```python
from build123d import *

# Parameters (mm, degrees)
SKETCH1_W           = 59.6
SKETCH1_H           = 35.5
BOSS_EXTRUDE1_DEPTH = 2.5
SKETCH3_W           = 59.6
SKETCH3_H           = 35.5
SKETCH3_W_2         = 54.6
SKETCH3_H_2         = 30.5
BOSS_EXTRUDE4_DEPTH = 38.5
SKETCH4_W           = 3.2
SKETCH4_H           = 3.2
SKETCH4_R           = 0.5
BOSS_EXTRUDE7_DEPTH = 5
FILLET1_R           = 0.25
FILLET2_R           = 0.25
SKETCH6_R           = 2
CUT_EXTRUDE1_DEPTH  = 5
FILLET4_R           = 0.3


with BuildPart() as part:
    # Sketch1 → Boss-Extrude1 (new body)
    with BuildSketch(Plane(origin=(0, 0, 0), x_dir=(1, 0, 0), z_dir=(0, 1, 0))):
        Rectangle(SKETCH1_W, SKETCH1_H)
    extrude(amount=BOSS_EXTRUDE1_DEPTH)

    # Sketch3 → Boss-Extrude4 (add)
    with BuildSketch(Plane(origin=(0, 2.5, 0), x_dir=(1, 0, 0), z_dir=(0, 1, 0))):
        Rectangle(SKETCH3_W, SKETCH3_H)
        Rectangle(SKETCH3_W_2, SKETCH3_H_2, mode=Mode.SUBTRACT)
    extrude(amount=BOSS_EXTRUDE4_DEPTH)

    # Sketch4 → Boss-Extrude7 (add)
    # profile 1 of 4: a face of its own
    with BuildSketch(Plane(origin=(0, 41, 0), x_dir=(1, 0, 0), z_dir=(0, 1, 0))):
        with Locations((-25.7, 13.65)):
            Rectangle(SKETCH4_W, SKETCH4_H)
        with Locations(Location((-25.7, 13.65, 0), (0, 0, 270))):
            Circle(SKETCH4_R, mode=Mode.SUBTRACT)
    # profile 2 of 4: a face of its own
    with BuildSketch(Plane(origin=(0, 41, 0), x_dir=(1, 0, 0), z_dir=(0, 1, 0))):
        with Locations((25.7, 13.65)):
            Rectangle(SKETCH4_W, SKETCH4_H)
        with Locations(Location((25.7, 13.65, 0), (0, 0, 270))):
            Circle(SKETCH4_R, mode=Mode.SUBTRACT)
    # profile 3 of 4: a face of its own
    with BuildSketch(Plane(origin=(0, 41, 0), x_dir=(1, 0, 0), z_dir=(0, 1, 0))):
        with Locations((25.7, -13.65)):
            Rectangle(SKETCH4_W, SKETCH4_H)
        with Locations(Location((25.7, -13.65, 0), (0, 0, 270))):
            Circle(SKETCH4_R, mode=Mode.SUBTRACT)
    # profile 4 of 4: a face of its own
    with BuildSketch(Plane(origin=(0, 41, 0), x_dir=(1, 0, 0), z_dir=(0, 1, 0))):
        with Locations((-25.7, -13.65)):
            Rectangle(SKETCH4_W, SKETCH4_H)
        with Locations(Location((-25.7, -13.65, 0), (0, 0, 270))):
            Circle(SKETCH4_R, mode=Mode.SUBTRACT)
    extrude(amount=-BOSS_EXTRUDE7_DEPTH)

    # Fillet1
    fillet1_edges = [part.edges().sort_by_distance(p)[0] for p in [
        (-29.8, 20.5, -17.75),
        (-29.8, 20.5, 17.75),
        (29.8, 20.5, 17.75),
        (29.8, 20.5, -17.75),
    ]]
    fillet(fillet1_edges, radius=FILLET1_R)

    # Fillet2
    fillet2_edges = [part.edges().sort_by_distance(p)[0] for p in [
        (0, 2.5, -15.25),
        (-27.3, 19.25, -15.25),
        (27.3, 19.25, -15.25),
        (27.3, 19.25, 15.25),
        (-27.3, 19.25, 15.25),
    ]]
    fillet(fillet2_edges, radius=FILLET2_R)

    # Sketch6 → Cut-Extrude1 (cut)
    with BuildSketch(Plane.ZY.offset(29.8)):
        with Locations((5.5, 12)):
            Circle(SKETCH6_R)
    extrude(amount=-CUT_EXTRUDE1_DEPTH, mode=Mode.SUBTRACT)

    # Fillet4
    fillet4_edges = [part.edges().sort_by_distance(p)[0] for p in [
        (-29.8, 12, 3.5),
    ]]
    fillet(fillet4_edges, radius=FILLET4_R)


solid = part.part
```
Geometry: final body of the model. Coordinates: model frame, mm. A direction names the side the tool comes from. Round coordinates to 2 decimals unless told otherwise and drop trailing zeros. Loops run counter-clockwise (first coordinate to the right, second up) from the corner with the lowest first, then second, coordinate; pieces in that order, holes last.
Item 1: Line query: L1, parallel to X at y = 37.45, z = 13.65; L2, parallel to Z at x = 12, y = 5; L3, parallel to X at y = 6.5, z = -13.5. Output: solid intervals per line, ascending.
Checked values:
L1: x = -29.8 to -26.2, -25.2 to -24.1, 24.1 to 25.2, 26.2 to 29.8
L2: z = -17.75 to -15.25, 15.25 to 17.75
L3: x = -29.8 to -27.3, 27.3 to 29.8
Item 2: Section A-A, the plane x = -2.5. Output: boundary loops of the cut face in (y, z).
Checked values:
outline: (0, -17.75) - (41, -17.75) - (41, -15.25) - (2.75, -15.25) arc R0.25 cw to (2.5, -15) - (2.5, 15.25) - (41, 15.25) - (41, 17.75) - (0, 17.75) - close
Item 3: Section B-B, the plane y = 7. Output: boundary loops of the cut face in (x, z).
Checked values:
outline: (-29.8, -17.5) arc R0.25 ccw to (-29.55, -17.75) - (29.55, -17.75) arc R0.25 ccw to (29.8, -17.5) - (29.8, 17.5) arc R0.25 ccw to (29.55, 17.75) - (-29.55, 17.75) arc R0.25 ccw to (-29.8, 17.5) - close; hole (-27.3, -15) arc R0.25 ccw to (-27.05, -15.25) - (27.05, -15.25) arc R0.25 ccw to (27.3, -15) - (27.3, 15) arc R0.25 ccw to (27.05, 15.25) - (-27.05, 15.25) arc R0.25 ccw to (-27.3, 15) - close
Item 4: Mould query, pull axis Z, two halves, no side actions, for faces 6 (the flat face through (0, 41, -16)), 7 (the flat face through (26, 39, -12.05)), 8 (the flat face through (0, 20, 17.75)). Classes: released by +Z, released by -Z, zero draft, split by the parting line, or undercut.
Checked values:
face 6: zero draft
face 7: undercut
face 8: released by +Z
Item 5: Section D-D, the plane y = 12. Output: boundary loops of the cut face in (x, z).
Checked values:
outline: (-29.8, -17.5) arc R0.25 ccw to (-29.55, -17.75) - (29.55, -17.75) arc R0.25 ccw to (29.8, -17.5) - (29.8, 17.5) arc R0.25 ccw to (29.55, 17.75) - (-29.55, 17.75) arc R0.25 ccw to (-29.8, 17.5) - (-29.8, 7.8) arc R0.3 ccw to (-29.5, 7.5) - (-27.3, 7.5) - (-27.3, 15) arc R0.25 cw to (-27.05, 15.25) - (27.05, 15.25) arc R0.25 cw to (27.3, 15) - (27.3, -15) arc R0.25 cw to (27.05, -15.25) - (-27.05, -15.25) arc R0.25 cw to (-27.3, -15) - (-27.3, 3.5) - (-29.5, 3.5) arc R0.3 ccw to (-29.8, 3.2) - close
Item 6: Reachability of faces 1 (the flat face through (29.8, 20, 0)), 2 (the flat face through (-24.1, 39, -14)), 3 (the flat face through (25, 36, -14)), 4 (the flat face through (-29.8, 20, 0)), 5 (the cylindrical face through (-28.415, 13.983, 5.24)) from +Z, -Z, +X, -X, +Y, -Y: full face, straight path, thin tool, end or side. Return the list, or none.
Checked values:
face 1: +Z, -Z, +X, +Y, -Y
face 2: +Y
face 3: none
face 4: +Z, -Z, -X, +Y, -Y
face 5: -X
Item 7: Contact query for a flat-ended pin moving along its axis: P1, Ø3, axis at x = 7, z = 7.5, coming from the +Y side. Output: stop coordinate, or through.
Checked values:
P1: stops at y = 2.5
Item 8: Section C-C, the plane z = 10. Output: boundary loops of the cut face in (x, y).
Checked values:
outline: (-29.8, 0) - (29.8, 0) - (29.8, 41) - (27.3, 41) - (27.3, 2.5) - (-27.3, 2.5) - (-27.3, 41) - (-29.8, 41) - close
